Geometry check sheet. Reference: drawing and pictorial views, mm from the part's lowest x, y, z. A direction names the side the tool comes from. Round coordinates to 2 decimals unless told otherwise and drop trailing zeros. Order: outer loops, then holes, each group sorted by start corner. A loop starts at its lowest first (then second) coordinate and runs counter-clockwise, first axis right, second up. Notation, with made-up numbers: (-3.75, 21) -> (40.25, 21) arc R9 ccw to (40.25, 33) -> close; hole circle Ø8 at (87.5, 38.5). An arc over 180 degrees is marked (long way). Return JSON: item names as keys, results as strings. Group by question number.
1) Section check C-C on z = 6.75. Enter the section's corners in (x, y), plus the area to 3 significant figures.
2) Tool access check on the marked faces 1, 2 and 3. Record the directions out of +Z, -Z, +X, -X, +Y, -Y that give a thin tool (end or side, any length) a straight path to the whole face; none if there is none.
3) Section check A-A on z = 19. Enter the section's corners in (x, y).
4) Section check B-B on x = 3.5. Enter the section's corners in (y, z), plus the area to 3 significant figures.
5) Scan lines: L1, parallel to Y at x = 18.75, z = 15.5; L2, parallel to Z at x = 2.5, y = 2.5; L3, parallel to X at y = 4.25, z = 15.75. Record each from-to range of solid material in increasing order.
6) Depth check by flat-ended pin: pin 1 (1.6 mm diameter, centred on x = 26.5, z = 3, fed in from +Y) (1 decimal); pin 2 (2 mm diameter, centred on y = 4, z = 11.5, fed in from +X); pin 3 (0.9 mm diameter, centred on x = 2.5, y = 3.5, fed in from +Z); pin 4 (1.5 mm diameter, centred on x = 3, y = 3, fed in from -Z). Enter the tip coordinate at first touch or a pass-through.
7) Section check D-D on x = 26.5. Enter the section's corners in (y, z).
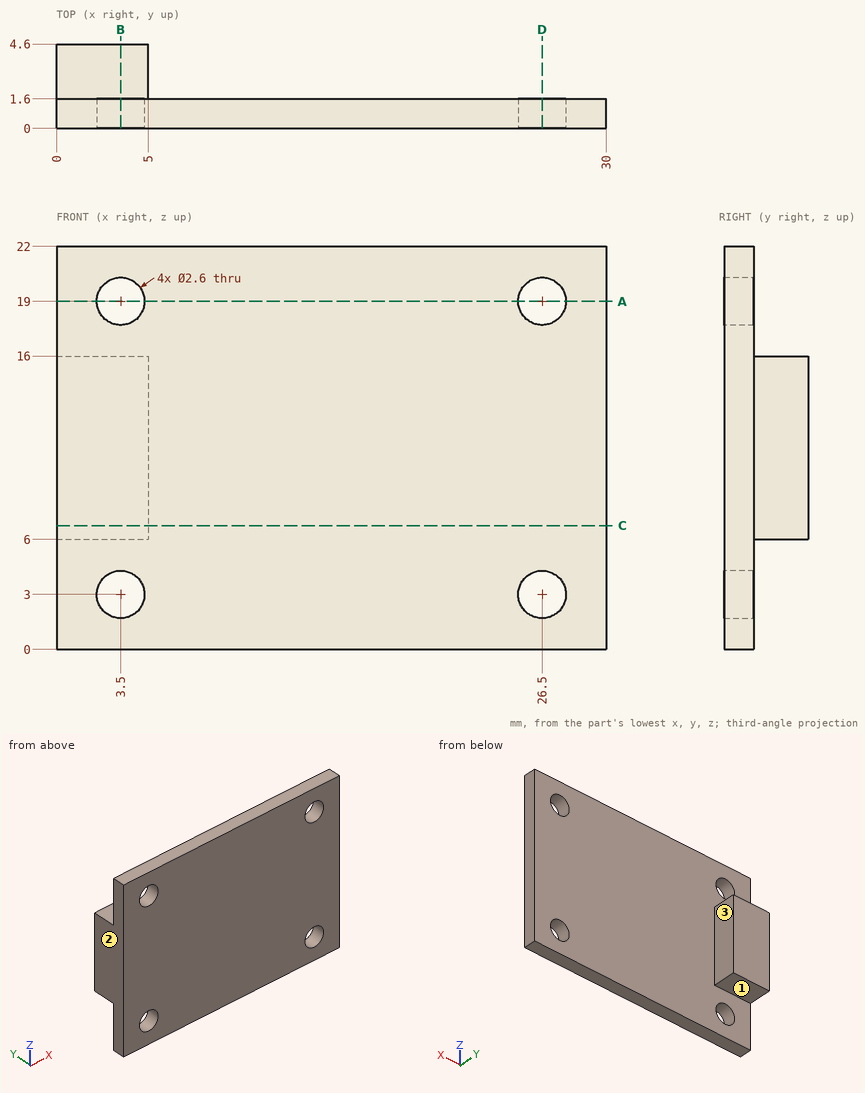
Check result:
{
 "1": {"outline": "(0, 0) -> (30, 0) -> (30, 1.6) -> (5, 1.6) -> (5, 4.6) -> (0, 4.6) -> close", "area": "63.0 mm^2"},
 "2": {"face 1": "-Z, +X, -X, +Y", "face 2": "+Z, -Z, -X, +Y, -Y", "face 3": "+Z, -Z, +X, +Y"},
 "3": {"outline": "(0, 0) -> (2.2, 0) -> (2.2, 1.6) -> (0, 1.6) -> close; (4.8, 0) -> (25.2, 0) -> (25.2, 1.6) -> (4.8, 1.6) -> close; (27.8, 0) -> (30, 0) -> (30, 1.6) -> (27.8, 1.6) -> close"},
 "4": {"outline": "(0, 0) -> (1.6, 0) -> (1.6, 1.7) -> (0, 1.7) -> close; (0, 4.3) -> (1.6, 4.3) -> (1.6, 6) -> (4.6, 6) -> (4.6, 16) -> (1.6, 16) -> (1.6, 17.7) -> (0, 17.7) -> close; (0, 20.3) -> (1.6, 20.3) -> (1.6, 22) -> (0, 22) -> close", "area": "56.9 mm^2"},
 "5": {"L1": "0 to 1.6", "L2": "6 to 16", "L3": "0 to 5"},
 "6": {"pin 1": "through", "pin 2": "x = 5", "pin 3": "z = 16", "pin 4": "z = 6"},
 "7": {"outline": "(0, 0) -> (1.6, 0) -> (1.6, 1.7) -> (0, 1.7) -> close; (0, 4.3) -> (1.6, 4.3) -> (1.6, 17.7) -> (0, 17.7) -> close; (0, 20.3) -> (1.6, 20.3) -> (1.6, 22) -> (0, 22) -> close"}
}
